```python
from build123d import *

# Parameters (mm, degrees)
CROQUIS1_R              = 2
SALIENTE_EXTRUIR1_DEPTH = 8
CORTAR_EXTRUIR1_DEPTH   = 3


with BuildPart() as part:
    # Croquis1 → Saliente-Extruir1 (new body)
    with BuildSketch(Plane.XY):
        with BuildLine():
            Line((0, 0), (-6.732907314, 0))
            Line((-6.732907314, 0), (-3.931702166, 6.415079868))
            ThreePointArc((-3.931702166, 6.415079868), (0, 8.988455594), (3.931702166, 6.415079868))
            Line((3.931702166, 6.415079868), (6.732907314, 0))
            Line((6.732907314, 0), (0, 0))
        make_face()
        with Locations((0.075747875, 5)):
            Circle(CROQUIS1_R, mode=Mode.SUBTRACT)
    extrude(amount=SALIENTE_EXTRUIR1_DEPTH)

    # Croquis2 → Cortar-Extruir1 (cut)
    with BuildSketch(Plane.XY.offset(8)):
        Polygon((-1.960251802, 1.508862843), (2.081161502, 1.491203979), (4.11716118, 4.982341136), (2.111747552, 8.491137157), (-1.929665752, 8.508796021), (-3.965665429, 5.017658864), align=None)
    extrude(amount=-CORTAR_EXTRUIR1_DEPTH, mode=Mode.SUBTRACT)


solid = part.part
```
Check sheet for the modelled part. Datum: model origin and axes. Units: mm. A direction names the side the tool comes from. Round coordinates to 2 decimals unless told otherwise and drop trailing zeros. Write each loop counter-clockwise with the first axis right and the second up, starting at its lowest first coordinate (ties: lowest second). Pieces come first, ordered by that corner, then holes. Notation, with made-up numbers: M 68,34 L 124,34 A25 cw 124,50 Z; hole C 77.5,88 d6. An arc over 180 degrees is marked long. Write item = value, one per line. Start each with the question number.
1. Gauge pin test, flat ends, axial feed: pin 1 (3.5 mm diameter, centred on x = 0.08, y = 5, fed in from -Z); pin 2 (3 mm diameter, centred on x = -2, z = 3.5, fed in from +Y); pin 3 (1 mm diameter, centred on y = 3, z = 6.5, fed in from +X); pin 4 (3 mm diameter, centred on y = 4.5, z = 5.5, fed in from -X). Record the tip position at first contact, or that the pin passes through.
2. Scan lines: line 1 (X direction, y = 3.75, z = 2); line 2 (X direction, y = 5, z = 3.4); line 3 (Z direction, x = 2, y = 2). Record each from-to range of solid material in increasing order. Write a range as [from, to].
3. Release check for a two-part mould opening along X. For faces 3 (the cylindrical face through (-0.07, 8.988, 3.944)), 4 (the flat face through (0, 0, 4)), 5 (the flat face through (-5.352, 3.163, 3.944)), 6 (the flat face through (-2.98, 3.29, 6.52)) record: pulls with the +X half, pulls with the -X half, needs draft (parallel to the pull), parting line crosses it, or undercut.
4. Section check D-D, the plane x = -3.5. Record the cut outline in (y, z).
5. Section check A-A, the plane z = 4.75. Record the cut outline in (x, y), then the cut area to 3 significant figures.
6. Tool access check on faces 1 (the flat face through (0.1, 2.6, 0)), 2 (the flat face through (-2.93, 6.79, 6.52)). Record the directions out of +Z, -Z, +X, -X, +Y, -Y that give a thin tool (end or side, any length) a straight path to the whole face; none if there is none.
7. Section check C-C, the plane y = 7.75. Record the cut outline in (x, z).
8. Section check B-B, the plane y = 3.25. Record the cut outline in (x, z), then the cut area to 3 significant figures.
Results found:
q1.pin_1 = through
q1.pin_2 = 8.96
q1.pin_3 = 5.64
q1.pin_4 = -5.42
q2.line_1 = [-5.1, -1.49], [1.64, 5.1]
q2.line_2 = [-4.55, -1.92], [2.08, 4.55]
q2.line_3 = [0, 5]
q3.face_3 = parting line crosses it
q3.face_4 = needs draft
q3.face_5 = pulls with the -X half
q3.face_6 = undercut
q4.outline = M 0,0 L 7.18,0 L 7.18,8 L 5.82,8 L 5.82,5 L 4.2,5 L 4.2,8 L 0,8 Z
q5.outline = M -6.73,0 L 6.73,0 L 3.93,6.42 A4.29 ccw -3.93,6.42 Z; hole C 0.08,5 d4
q5.area = 70.4 mm^2
q6.face_1 = -Z, +X, -X, +Y, -Y
q6.face_2 = +Z
q7.outline = M -3.02,0 L 3.02,0 L 3.02,8 L 2.54,8 L 2.54,5 L -2.37,5 L -2.37,8 L -3.02,8 Z
q8.outline = M -5.31,0 L -0.89,0 L -0.89,5 L -2.96,5 L -2.96,8 L -5.31,8 Z; M 1.04,0 L 5.31,0 L 5.31,8 L 3.11,8 L 3.11,5 L 1.04,5 Z
q8.area = 57.2 mm^2
